Check sheet for the modelled part. Datum: model origin and axes. Units: mm. A direction names the side the tool comes from. Round coordinates to 2 decimals unless told otherwise and drop trailing zeros. Order: outer loops, then holes, each group sorted by start corner. A loop starts at its lowest first (then second) coordinate and runs counter-clockwise, first axis right, second up.
Q1. Cross-section at C-C on y = 7.5. Record the cut outline in (x, z), then the cut area to 3 significant figures.
Q2. Mould release check, pull along X, two halves, no side actions. Record for faces 1 (the flat face through (0, 10, 98)), 2 (the flat face through (19.05, 10, 98)), 3 (the flat face through (9, 10, 0)), 4 (the flat face through (7.5, 14.884, 173.2)): +X half, -X half, draft (parallel to the pull), parting line (faces both ways), or undercut.
Q3. Depth check by flat-ended pin: P1, Ø5, axis at x = 14, y = 9, coming from the -Z side; P2, Ø6, axis at x = 9.5, y = 10, coming from the +Z side; P3, Ø2, axis at x = 15, y = 8, coming from the +Z side. Enter the tip coordinate at first touch or a pass-through.
Q4. Set-up check for faces 5 (the cylindrical face through (9.411, 16.996, 167.485)), 6 (the flat face through (10, 19.05, 94)): record each of +Z, -Z, +X, -X, +Y, -Y from which the full face is reachable in a straight line by a thin tool's end or side.
Q5. Cross-section at B-B on x = 15.5. Record the cut outline in (y, z), then the cut area to 3 significant figures.
Q6. Cross-section at A-A on z = 171.45. Record the cut outline in (x, y).
Q7. Scan lines: probe 1 along X at (y, z) = (16.55, 171.45); probe 2 along Z at (x, y) = (10, 12); probe 3 along X at (y, z) = (3.75, 171.45). Record each from-to range of solid material in increasing order.
from build123d import *

# Parameters (mm, degrees)
SKETCH1_W                                      = 19.05
SKETCH1_H                                      = 19.05
BOSS_EXTRUDE1_DEPTH                            = 177.8
BOSS_EXTRUDE2_DEPTH                            = 19.05
CBORE_FOR_8_SOCKET_HEAD_CAP_SCREW1_D           = 4.3053
CBORE_FOR_8_SOCKET_HEAD_CAP_SCREW1_DEPTH       = 19.05
CBORE_FOR_8_SOCKET_HEAD_CAP_SCREW1_CBORE_D     = 7.9375
CBORE_FOR_8_SOCKET_HEAD_CAP_SCREW1_CBORE_DEPTH = 4.1656


with BuildPart() as part:
    # Sketch1 → Boss-Extrude1 (new body)
    with BuildSketch(Plane.XY):
        with Locations((9.525, 9.525)):
            Rectangle(SKETCH1_W, SKETCH1_H)
    extrude(amount=BOSS_EXTRUDE1_DEPTH)

    # Sketch2 → Boss-Extrude2 (add)
    with BuildSketch(Plane(origin=(19.05, 0, 0), x_dir=(0, 0, -1), z_dir=(1, 0, 0))):
        with BuildLine():
            Line((-177.8, 19.05), (-190.5, 19.05))
            ThreePointArc((-190.5, 19.05), (-192.843013973, 17.490757626), (-192.309392774, 14.727390174))
            Line((-192.309392774, 14.727390174), (-177.8, 0))
            Line((-177.8, 0), (-177.8, 19.05))
        make_face()
    extrude(amount=-BOSS_EXTRUDE2_DEPTH)

    # CBORE for #8 Socket Head Cap Screw1
    with Locations(Plane(origin=(9.23608704, 19.05, 171.45), x_dir=(0, 0, 1), z_dir=(0, 1, 0))):
        with Locations((0, 0)):
            CounterBoreHole(CBORE_FOR_8_SOCKET_HEAD_CAP_SCREW1_D / 2, CBORE_FOR_8_SOCKET_HEAD_CAP_SCREW1_CBORE_D / 2, CBORE_FOR_8_SOCKET_HEAD_CAP_SCREW1_CBORE_DEPTH, depth=CBORE_FOR_8_SOCKET_HEAD_CAP_SCREW1_DEPTH)


solid = part.part
Results found:
1. outline: (0, 0) - (19.05, 0) - (19.05, 185.19) - (0, 185.19) - close; hole circle Ø4.31 at (9.24, 171.45)
1. area: 3,510 mm2
2. face 1: -X half
2. face 2: +X half
2. face 3: draft
2. face 4: undercut
3. P1: stops at z = 0
3. P2: stops at z = 190.61
3. P3: stops at z = 186.67
4. face 5: +Y
4. face 6: +Z, -Z, +X, -X, +Y
5. outline: (0, 0) - (19.05, 0) - (19.05, 190.5) arc R2.54 ccw to (14.73, 192.31) - (0, 177.8) - close
5. area: 3,560 mm2
6. outline: (0, 0) - (7.08, 0) - (7.08, 14.88) - (5.27, 14.88) - (5.27, 19.05) - (0, 19.05) - close; (11.39, 0) - (19.05, 0) - (19.05, 19.05) - (13.2, 19.05) - (13.2, 14.88) - (11.39, 14.88) - close
7. probe 1: x = 0 to 5.27, 13.2 to 19.05
7. probe 2: z = 0 to 169.44, 173.46 to 189.62
7. probe 3: x = 0 to 7.08, 11.39 to 19.05
